Autodesk Inventor part; units mm, degrees
ref_plane "YZ Plane" through (0, 0, 0) normal (1, 0, 0) x (0, 1, 0)
ref_plane "XZ Plane" through (0, 0, 0) normal (0, 1, 0) x (-1, 0, 0)
ref_plane "XY Plane" through (0, 0, 0) normal (0, 0, 1) x (1, 0, 0)
sketch "スケッチ1" plane through (0, 0, 0) normal (0, 0, 1) x (1, 0, 0)
  line L0 (0, 0) -> (9, 0)
  line L1 (9, 0) -> (9, -9)
  line L2 (9, -9) -> (0, -9)
  line L3 (0, -9) -> (0, 0)
  line L4 (1.2, -7.8) -> (7.8, -7.8)
  line L5 (7.8, -7.8) -> (7.8, -1.2)
  line L6 (7.8, -1.2) -> (1.2, -1.2)
  line L7 (1.2, -1.2) -> (1.2, -7.8)
  dimension "d0" = 9
  dimension "d1" = 9
  dimension "d2" = 6.6
  dimension "d3" = 6.6
  dimension "d4" = 1.2
  dimension "d5" = 1.2
extrude "押し出し1" add sketch "スケッチ1" along normal blind 74
sketch "スケッチ2" plane through (0, 0, 0) normal (0, 1, 0) x (1, 0, 0)
  line L0 (9, -74) -> (0, -74)
  line L1 (9, 0) -> (0, 0)
  line L2 (0, 0) -> (0, -74)
  point P0 (4.5, -69.5)
  point P1 (4.5, -4.5)
  dimension "d8" = 4.5
  dimension "d9" = 4.5
  dimension "d10" = 4.5
  dimension "d11" = 4.5
hole "穴1" at (4.5, 0, 69.5) at (4.5, 0, 4.5) direction (0, -1, 0) diameter 3 end through all
sketch "スケッチ3" plane through (0, -9, 0) normal (-1, 0, 0) x (0, 0, 1)
  line L0 (0, 9) -> (0, 0)
  line L1 (74, 9) -> (74, 0)
  line L2 (0, 0) -> (74, 0)
  point P0 (60.5, 4.5)
  point P1 (13.5, 4.5)
  dimension "d19" = 13.5
  dimension "d20" = 13.5
  dimension "d21" = 4.5
  dimension "d22" = 4.5
hole "穴2" at (0, -4.5, 60.5) at (0, -4.5, 13.5) direction (1, 0, 0) diameter 3 end through all
sketch "スケッチ4" plane through (0, 0, 0) normal (0, 1, 0) x (1, 0, 0)
  circle A0 centre (4.5, -4.5) radius 1.5
  circle A1 centre (4.5, -69.5) radius 1.5
  circle A2 centre (4.5, -69.5) radius 1.5
  line L0 (4.5, -69.5) -> (4.5, -4.5)
  point P0 (0, 0)
  point P1 (4.5, -63)
  point P2 (4.5, -56.5)
  point P3 (4.5, -50)
  point P4 (4.5, -43.5)
  point P5 (4.5, -37)
  point P6 (4.5, -30.5)
  point P7 (4.5, -24)
  point P8 (4.5, -17.5)
  point P9 (4.5, -11)
  dimension "d30" = 65
  dimension "d31" = 6.5
  dimension "d34" = 6.5
hole "穴3" at (4.5, 0, 63) at (4.5, 0, 56.5) at (4.5, 0, 50) at (4.5, 0, 43.5) at (4.5, 0, 37) at (4.5, 0, 30.5) at (4.5, 0, 24) at (4.5, 0, 17.5) at (4.5, 0, 11) direction (0, -1, 0) diameter 5.5 end through all
sketch "スケッチ5" plane through (0, -9, 0) normal (-1, 0, 0) x (0, 0, 1)
  line L0 (74, 9) -> (74, 0)
  line L1 (0, 9) -> (0, 0)
  line L2 (0, 0) -> (74, 0)
  circle A0 centre (60.5, 4.5) radius 1.5
  circle A1 centre (13.5, 4.5) radius 1.5
  line L3 (60.5, 4.5) -> (13.5, 4.5)
  point P0 (67.25, 4.5)
  point P1 (6.75, 4.5)
  point P2 (53.7857, 4.5)
  point P3 (47.0714, 4.5)
  point P4 (40.3571, 4.5)
  point P5 (33.6429, 4.5)
  point P6 (26.9286, 4.5)
  point P7 (20.2143, 4.5)
  dimension "d46" = 6.75
  dimension "d47" = 6.75
  dimension "d48" = 4.5
  dimension "d49" = 4.5
  dimension "d50" = 47
  dimension "d51" = 6.7143
  dimension "d54" = 6.7143
hole "穴4" at (0, -4.5, 67.25) at (0, -4.5, 6.75) at (0, -4.5, 53.7857) at (0, -4.5, 47.0714) at (0, -4.5, 40.3571) at (0, -4.5, 33.6429) at (0, -4.5, 26.9286) at (0, -4.5, 20.2143) direction (1, 0, 0) diameter 5.5 end through all
properties part number "ロボット回転9x9_4" material "アルミニウム 6061"
The model under review builds one solid part; all positions refer to its coordinate system, in mm. A direction names the side the tool comes from. Round coordinates to 2 decimals unless told otherwise and drop trailing zeros. Order: outer loops, then holes, each group sorted by start corner. A loop starts at its lowest first (then second) coordinate and runs counter-clockwise, first axis right, second up. Notation, with made-up numbers: (-7.75, 61) -> (30.25, 61) arc R6 cw to (30.25, 72) -> close; hole circle Ø7 at (-2.5, -37). An arc over 180 degrees is marked (long way). Use a Markdown table: item, result.
Q1. Tool access review of faces 3 (the cylindrical face through (4.379, -0.608, 34.253)), 4 (the flat face through (7.5, -1.2, 36.5)): name each direction out of +Z, -Z, +X, -X, +Y, -Y from which nothing blocks a thin tool from reaching the whole face with its end or side.
Values:
| item | result |
|---|---|
| face 3 | +Y, -Y |
| face 4 | +Z, -Z |
Q2. Clearance check with a flat-ended pin moving along its axis: P1, Ø5, axis at x = 4.5, y = -2.5, coming from the +Z side. State where the tip first meets the part, or that it passes through.
Values:
| item | result |
|---|---|
| P1 | stops at z = 74 |
Q3. For line 1 (X direction, y = -6, z = 4); line 2 (X direction, y = -8.35, z = 43.5); line 3 (Y direction, x = 4.75, z = 40.5), list the stretches that pass through material, from the lowest coordinate up.
Values:
| item | result |
|---|---|
| line 1 | x = 0 to 1.2, 7.8 to 9 |
| line 2 | x = 0 to 1.75, 7.25 to 9 |
| line 3 | y = -9 to -7.8, -1.2 to 0 |
Q4. We need section B-B on y = -4.5. State how many separate pieces and enclosed holes the cut face has, then the cut area to 3 significant figures.
Values:
| item | result |
|---|---|
| separate pieces | 22 |
| enclosed holes | 0 |
| area | 57.6 mm^2 |
Q5. Mouldability with a two-part tool opening along Y and no side actions: class faces 1 (the cylindrical face through (4.379, -0.608, 27.753)), 2 (the cylindrical face through (8.41, -3.45, 42.9)) as +Y half, -Y half, draft (parallel to the pull), parting line (faces both ways), or undercut.
Values:
| item | result |
|---|---|
| face 1 | draft |
| face 2 | undercut |
Q6. We need section A-A on z = 6.75. Write out the cut boundary in (x, y).
Values:
| item | result |
|---|---|
| outline | (0, -9) -> (9, -9) -> (9, -7.25) -> (7.8, -7.25) -> (7.8, -7.8) -> (1.2, -7.8) -> (1.2, -7.25) -> (0, -7.25) -> close; (0, -1.75) -> (1.2, -1.75) -> (1.2, -1.2) -> (7.8, -1.2) -> (7.8, -1.75) -> (9, -1.75) -> (9, 0) -> (0, 0) -> close |
Q7. We need section C-C on z = 39. Write out the cut boundary in (x, y).
Values:
| item | result |
|---|---|
| outline | (0, -9) -> (2.61, -9) -> (2.61, -7.8) -> (1.2, -7.8) -> (1.2, -6.89) -> (0, -6.89) -> close; (0, -2.11) -> (1.2, -2.11) -> (1.2, -1.2) -> (2.61, -1.2) -> (2.61, 0) -> (0, 0) -> close; (6.39, -9) -> (9, -9) -> (9, -6.89) -> (7.8, -6.89) -> (7.8, -7.8) -> (6.39, -7.8) -> close; (6.39, -1.2) -> (7.8, -1.2) -> (7.8, -2.11) -> (9, -2.11) -> (9, 0) -> (6.39, 0) -> close |
